Design review of the part built by this model. Coordinates are the model's own, in mm. Face numbers are marked on the shaded views. A direction names the side the tool comes from. Coordinates: 2 decimals unless noted, no trailing zeros. Loops run counter-clockwise (first coordinate to the right, second up) from the corner with the lowest first, then second, coordinate; pieces in that order, holes last. Notation, with made-up numbers: (-32.5, 2.5) -> (-28.5, 2.5) arc R17 cw to (-28.5, 20.5) -> close; hole circle Ø6 at (-21.5, 18). An arc over 180 degrees is marked (long way). One line per item, written item: value. Start each with the question number.
1. Machinability: for the marked faces 3, 4 and 5, which of the approach directions +Z, -Z, +X, -X, +Y, -Y give a long, thin tool a straight path to every point of the face, cutting with its end or side? Answer none if there is none.
2. Add section B-B on z = 1.25. Write out the cut boundary in (x, y), plus the area to 3 significant figures.
3. Draft analysis for pull direction X (two halves, no side actions). For the marked faces 1 and 2, state which applies: pulls with the +X half, pulls with the -X half, needs draft (parallel to the pull), parting line crosses it, or undercut.
4. For probe 1 along Y at (x, z) = (15, 1.35); probe 2 along Z at (x, y) = (-2, -3); probe 3 along X at (y, z) = (-0.5, -0.75), list the stretches that pass through material, from the lowest coordinate up.
5. Add section A-A on x = 15. Write out the cut boundary in (y, z).
6. Add section D-D on z = -10. Write out the cut boundary in (x, y), plus the area to 3 significant figures.
7. Insertion check: pin 1 (1 mm diameter, centred on x = 17, z = 1.5, fed in from +Y); pin 2 (5 mm diameter, centred on x = 19.5, y = -0.5, fed in from -Z); pin 3 (3 mm diameter, centred on y = -1, z = -3, fed in from +X). Each pin has a flat end and moves straight along its axis. Give the tip position at first contact, or say it passes through.
```python
from build123d import *

# Parameters (mm, degrees)
F1_DEPTH = 2
F2_R     = 2.5
F3_DEPTH = 2
F4_R     = 2
F5_DEPTH = 7
F6_R     = 1.5
F7_DEPTH = 11
F8_D     = 4


# Not quite as in the source:
# - a feature names something its author has since deleted; it is built from what else it names


with BuildPart() as f1:
    # F0 (on Top) → F1 (new body)
    with BuildSketch(Plane.XY):
        with BuildLine():
            ThreePointArc((4.4790320824, 2.2222222222), (-4.249182928, 2.6352313835), (0, -5))
            Line((0, -5), (30, -5))
            ThreePointArc((30, -5), (34.249182928, 2.6352313835), (25.5209679176, 2.2222222222))
            ThreePointArc((25.5209679176, 2.2222222222), (24.0459273585, 0.6006536576), (21.9377422517, 0))
            Line((21.9377422517, 0), (21.6697930593, 0))
            ThreePointArc((21.6697930593, 0), (21.1697930593, 0.1339745962), (20.8037676555, 0.5))
            Line((20.8037676555, 0.5), (20.2264173863, 1.5))
            ThreePointArc((20.2264173863, 1.5), (19.8603919825, 1.8660254038), (19.3603919825, 2))
            Line((19.3603919825, 2), (10.6396080175, 2))
            ThreePointArc((10.6396080175, 2), (10.1396080175, 1.8660254038), (9.7735826137, 1.5))
            Line((9.7735826137, 1.5), (9.1962323445, 0.5))
            ThreePointArc((9.1962323445, 0.5), (8.8302069407, 0.1339745962), (8.3302069407, 0))
            Line((8.3302069407, 0), (8.0622577483, 0))
            ThreePointArc((8.0622577483, 0), (5.9540726415, 0.6006536576), (4.4790320824, 2.2222222222))
        make_face()
    extrude(amount=F1_DEPTH)

    # F2 (on Top) → F3 (join)
    with BuildSketch(Plane.XY):
        Circle(F2_R)
        with Locations((30, 0)):
            Circle(F2_R)
    extrude(amount=-F3_DEPTH)

    # F4 (on Top) → F5 (join)
    with BuildSketch(Plane.XY):
        Circle(F4_R)
        with Locations((30, 0)):
            Circle(F4_R)
    extrude(amount=-F5_DEPTH)

    # F6 (on Top) → F7 (join)
    with BuildSketch(Plane.XY):
        Circle(F6_R)
        with Locations((30, 0)):
            Circle(F6_R)
    extrude(amount=-F7_DEPTH)

    # F8 (through all)
    with Locations(Plane(origin=(0, 0, 0), x_dir=(1, 0, 0), z_dir=(0, 0, -1))):
        with Locations((15, 1.5)):
            Hole(F8_D / 2)


solid = f1.part
```
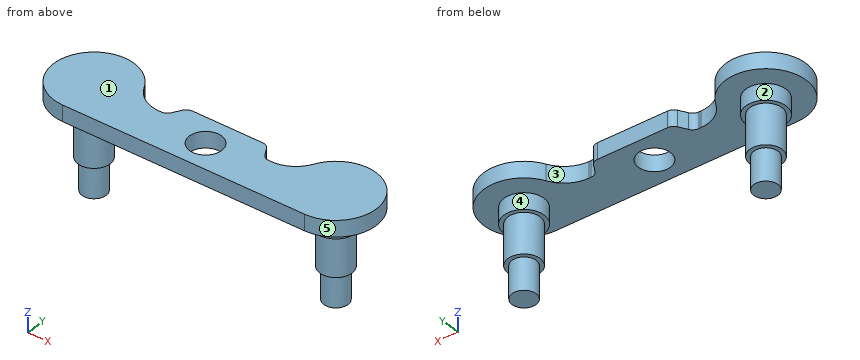
Worked answers:
1. face 3: +Z, -Z, +Y
1. face 4: -Z
1. face 5: +Z, -Z
2. outline: (0, -5) -> (30, -5) arc R5 ccw (long way) to (25.52, 2.22) arc R4 cw to (21.94, 0) -> (21.67, 0) arc R1 cw to (20.8, 0.5) -> (20.23, 1.5) arc R1 ccw to (19.36, 2) -> (10.64, 2) arc R1 ccw to (9.77, 1.5) -> (9.2, 0.5) arc R1 cw to (8.33, 0) -> (8.06, 0) arc R4 cw to (4.48, 2.22) arc R5 ccw (long way) to start; hole circle Ø4 at (15, -1.5)
2. area: 280 mm²
3. face 1: needs draft
3. face 2: undercut
4. probe 1: y = -5 to -3.5, 0.5 to 2
4. probe 2: z = 0 to 2
4. probe 3: x = -2.45 to 2.45, 27.55 to 32.45
5. outline: (-5, 0) -> (-3.5, 0) -> (-3.5, 2) -> (-5, 2) -> close; (0.5, 0) -> (2, 0) -> (2, 2) -> (0.5, 2) -> close
6. outline: circle Ø3 at (0, 0); circle Ø3 at (30, 0)
6. area: 14.1 mm²
7. pin 1: stops at y = 2
7. pin 2: stops at z = 0
7. pin 3: stops at x = 32.5
